Model file for the job. Use its own axes, mm. Round coordinates to 2 decimals unless told otherwise and drop trailing zeros. Loops run counter-clockwise (first coordinate to the right, second up) from the corner with the lowest first, then second, coordinate; pieces in that order, holes last. Notation, with made-up numbers: (18, -12.75) - (74, -12.75) arc R15 ccw to (74, -5.75) - close; hole circle Ø9 at (-1.5, -18). An arc over 180 degrees is marked (long way). Answer as a JSON object with one key per item and string values.
from build123d import *

# Parameters (mm, degrees)
BOSS_EXTRUDE1_DEPTH                                 = 1.75
CSK_FOR_M3_COUNTERSUNK_FLAT_HEAD_SCREW1_D           = 3.4
CSK_FOR_M3_COUNTERSUNK_FLAT_HEAD_SCREW1_DEPTH       = 3.5
CSK_FOR_M3_COUNTERSUNK_FLAT_HEAD_SCREW1_CSINK_D     = 6.3
CSK_FOR_M3_COUNTERSUNK_FLAT_HEAD_SCREW1_CSINK_ANGLE = 90
CSK_FOR_M3_COUNTERSUNK_FLAT_HEAD_SCREW1_TIP         = 1.021463052


with BuildPart() as part:
    # Sketch1 → Boss-Extrude1 (new, symmetric)
    with BuildSketch(Plane.XY):
        Polygon((2, -3.464101615), (4, 0), (2, 3.464101615), (-2, 3.464101615), (-4, 0), (-2, -3.464101615), align=None)
    extrude(amount=BOSS_EXTRUDE1_DEPTH, both=True)

    # CSK for M3 Countersunk Flat Head Screw1
    with Locations(Plane(origin=(0, 0, -1.75), x_dir=(-1, 0, 0), z_dir=(0, 0, -1))):
        with Locations((0, 0)):
            CounterSinkHole(CSK_FOR_M3_COUNTERSUNK_FLAT_HEAD_SCREW1_D / 2, CSK_FOR_M3_COUNTERSUNK_FLAT_HEAD_SCREW1_CSINK_D / 2, depth=CSK_FOR_M3_COUNTERSUNK_FLAT_HEAD_SCREW1_DEPTH, counter_sink_angle=CSK_FOR_M3_COUNTERSUNK_FLAT_HEAD_SCREW1_CSINK_ANGLE)
            with Locations((0, 0, -(CSK_FOR_M3_COUNTERSUNK_FLAT_HEAD_SCREW1_DEPTH + CSK_FOR_M3_COUNTERSUNK_FLAT_HEAD_SCREW1_TIP / 2))):  # 118° drill point
                Cone(0, CSK_FOR_M3_COUNTERSUNK_FLAT_HEAD_SCREW1_D / 2, CSK_FOR_M3_COUNTERSUNK_FLAT_HEAD_SCREW1_TIP, mode=Mode.SUBTRACT)


solid = part.part
1) Slice it at B-B on z = -0.1. List the corners of the cut face in (x, y).
Values follow:
{"outline": "(-4, 0) - (-2, -3.46) - (2, -3.46) - (4, 0) - (2, 3.46) - (-2, 3.46) - close; hole circle Ø3.4 at (0, 0)"}
2) Slice it at A-A on x = 0. List the corners of the cut face in (y, z).
Values follow:
{"outline": "(-3.46, -1.75) - (-3.15, -1.75) - (-1.7, -0.3) - (-1.7, 1.75) - (-3.46, 1.75) - close; (1.7, -0.3) - (3.15, -1.75) - (3.46, -1.75) - (3.46, 1.75) - (1.7, 1.75) - close"}
3) Two-plate mould, pull along Y, no slides. Class faces 1 (the cylindrical face through (-0.37, -1.66, 0.74)), 2 (the flat face through (3.014, 1.708, 0.024)), 3 (the flat face through (2, 0, 1.75)), 4 (the flat face through (0, -3.464, 0)): pulls with the +Y half, pulls with the -Y half, needs draft (parallel to the pull), parting line crosses it, or undercut.
Values follow:
{"face 1": "undercut", "face 2": "pulls with the +Y half", "face 3": "needs draft", "face 4": "pulls with the -Y half"}
4) Probe probe 1 along Y at (x, z) = (0, 0.7); probe 2 along Y at (x, z) = (-1.75, -0.75); probe 3 along X at (y, z) = (2, -1). List the from-to ranges inside material, lowest first.
Values follow:
{"probe 1": "-3.46 to -1.7, 1.7 to 3.46", "probe 2": "-3.46 to -1.25, 1.25 to 3.46", "probe 3": "-2.85 to -1.33, 1.33 to 2.85"}
5) Drop flat-ended pins along their axis: P1, Ø2, axis at y = 1.5, z = -1, coming from the -X side; P2, Ø2, axis at y = 1.5, z = 1, coming from the +X side; P3, Ø1.5, axis at y = -1.5, z = -1, coming from the +X side. Give the stop position or say it passes through.
Values follow:
{"P1": "x = -3.71", "P2": "x = 3.71", "P3": "x = 3.57"}
